Here's how the part is built. I have some questions about the finished solid (model axes, mm). Face numbers are marked on the shaded views. A direction names the side the tool comes from. Coordinates: 2 decimals unless noted, no trailing zeros. Write each loop counter-clockwise with the first axis right and the second up, starting at its lowest first coordinate (ties: lowest second). Pieces come first, ordered by that corner, then holes.
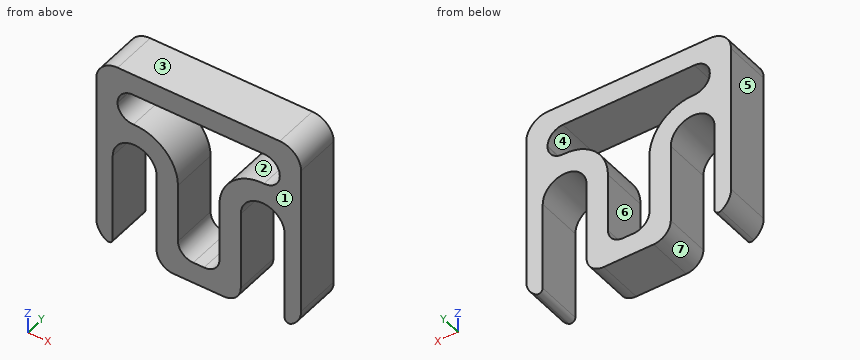
```python
from build123d import *

# Parameters (mm, degrees)
BOSS_EXTRUDE1_DEPTH     = 6.858
FILLET1_R               = 2.54
FILLET2_R               = 0.635
CUT_EXTRUDE1_DEPTH      = 308.470862171
CUT_EXTRUDE1_DEPTH_BACK = 308.470862171
FILLET3_R               = 2.286


with BuildPart() as part:
    # Sketch1 → Boss-Extrude1 (new body)
    with BuildSketch(Plane(origin=(0, 546.1, 533.938575125), x_dir=(1, 0, 0), z_dir=(0, -1, 0))):
        with BuildLine():
            Line((21.5011, -242.346575125), (21.5011, -256.634075125))
            Line((21.5011, -256.634075125), (8.9789, -256.634075125))
            Line((8.9789, -256.634075125), (8.9789, -242.346575125))
            ThreePointArc((8.9789, -242.346575125), (5.715, -239.082675125), (2.4511, -242.346575125))
            Line((2.4511, -242.346575125), (2.4511, -256.550449219))
            ThreePointArc((2.4511, -256.550449219), (0.687128671, -255.431667645), (0, -253.459075125))
            Line((0, -253.459075125), (0, -231.234075125))
            ThreePointArc((0, -231.234075125), (0.92993597, -228.989011095), (3.175, -228.059075125))
            Line((3.175, -228.059075125), (27.305, -228.059075125))
            ThreePointArc((27.305, -228.059075125), (29.55006403, -228.989011095), (30.48, -231.234075125))
            Line((30.48, -231.234075125), (30.48, -253.459075125))
            ThreePointArc((30.48, -253.459075125), (29.792871329, -255.431667645), (28.0289, -256.550449219))
            Line((28.0289, -256.550449219), (28.0289, -242.346575125))
            ThreePointArc((28.0289, -242.346575125), (24.765, -239.082675125), (21.5011, -242.346575125))
        make_face()
    extrude(amount=-BOSS_EXTRUDE1_DEPTH)

    # Fillet1
    fillet1_edges = [part.edges().sort_by_distance(p)[0] for p in [
        (21.5011, 549.529, 277.3045),
        (8.9789, 549.529, 277.3045),
    ]]
    fillet(fillet1_edges, radius=FILLET1_R)

    # Fillet2
    fillet2_edges = [part.edges().sort_by_distance(p)[0] for p in [
        (28.0289, 549.529, 277.388125906),
        (2.4511, 549.529, 277.388125906),
    ]]
    fillet(fillet2_edges, radius=FILLET2_R)

    # Sketch2 → Cut-Extrude1 (cut, two sides)
    with BuildSketch(Plane.XZ.offset(-546.1)) as cut_extrude1_sk:
        with BuildLine():
            Line((27.305, 297.508741773), (27.305, 302.7045))
            Line((27.305, 302.7045), (3.175, 302.7045))
            Line((3.175, 302.7045), (3.175, 297.508741773))
            ThreePointArc((3.175, 297.508741773), (9.257924442, 296.968534163), (12.1539, 291.592))
            Line((12.1539, 291.592), (12.1539, 280.4795))
            Line((12.1539, 280.4795), (18.3261, 280.4795))
            Line((18.3261, 280.4795), (18.3261, 291.592))
            ThreePointArc((18.3261, 291.592), (21.222075558, 296.968534163), (27.305, 297.508741773))
        make_face()
    extrude(amount=CUT_EXTRUDE1_DEPTH, mode=Mode.SUBTRACT)
    extrude(cut_extrude1_sk.sketch, amount=-CUT_EXTRUDE1_DEPTH_BACK, mode=Mode.SUBTRACT)

    # Fillet3
    fillet3_edges = [part.edges().sort_by_distance(p)[0] for p in [
        (27.305, 549.529, 297.508741773),
        (18.3261, 549.529, 280.4795),
        (12.1539, 549.529, 280.4795),
        (3.175, 549.529, 297.508741773),
        (3.175, 549.529, 302.7045),
        (27.305, 549.529, 302.7045),
    ]]
    fillet(fillet3_edges, radius=FILLET3_R)


solid = part.part
```
1) I need wall thicknesses on probe 1 along X at (y, z) = (547.75, 288.25); probe 2 along Z at (x, y) = (25, 551.25); probe 3 along X at (y, z) = (547.75, 280.75). Which ranges of each line are inside material? Lowest first, please.
Values follow:
probe 1: x = 0 to 2.45, 8.98 to 12.15, 18.33 to 21.5, 28.03 to 30.48
probe 2: z = 294.85 to 298.03, 302.7 to 305.88
probe 3: x = 0 to 2.45, 8.98 to 13.36, 17.12 to 21.5, 28.03 to 30.48
2) Imagine slicing it at B-B on x = 25.5. Please give me the cut outline in (y, z), then the cut area to 3 significant figures.
Values follow:
outline: (546.1, 294.77) - (552.96, 294.77) - (552.96, 298.08) - (546.1, 298.08) - close; (546.1, 302.65) - (552.96, 302.65) - (552.96, 305.88) - (546.1, 305.88) - close
area: 44.8 mm2
3) Imagine slicing it at C-C on z = 299.25. Please give me the cut outline in (x, y), then the cut area to 3 significant figures.
Values follow:
outline: (0, 546.1) - (3.44, 546.1) - (3.44, 552.96) - (0, 552.96) - close; (27.04, 546.1) - (30.48, 546.1) - (30.48, 552.96) - (27.04, 552.96) - close
area: 47.1 mm2
4) Will this pin go through, and if not, where does the flat tip stop? pin 1 (1.5 mm diameter, centred on x = 24, y = 547.5, fed in from -Z).
Values follow:
pin 1: stops at z = 294.48
5) We'd pull the mould along Z, two halves only. Please class the marked faces 1, 2, 3 and 4: pulls with the +Z half, pulls with the -Z half, needs draft (parallel to the pull), parting line crosses it, or undercut.
Values follow:
face 1: needs draft
face 2: undercut
face 3: pulls with the +Z half
face 4: undercut
6) On a 3-axis mill with a long thin cutter (end or side, diameter ignored), from which of +Z, -Z, +X, -X, +Y, -Y can I reach the whole of each face in a straight line? I mean the marked faces 5, 6 and 7. Say none if no direction works.
Values follow:
face 5: +Z, -Z, -X, +Y, -Y
face 6: +Y, -Y
face 7: -Z, +Y, -Y
7) Imagine slicing it at A-A on z = 287.5. Please give me the cut outline in (x, y), then the cut area to 3 significant figures.
Values follow:
outline: (0, 546.1) - (2.45, 546.1) - (2.45, 552.96) - (0, 552.96) - close; (8.98, 546.1) - (12.15, 546.1) - (12.15, 552.96) - (8.98, 552.96) - close; (18.33, 546.1) - (21.5, 546.1) - (21.5, 552.96) - (18.33, 552.96) - close; (28.03, 546.1) - (30.48, 546.1) - (30.48, 552.96) - (28.03, 552.96) - close
area: 77.2 mm2
